from build123d import *

# Parameters (mm, degrees)
F0_W           = 70
F0_H           = 120
F0_R           = 6.5
F0_R_2         = 13
F1_DEPTH       = 5
F3_D           = 4.4
F3_DEPTH       = 10
F3_CSINK_D     = 8.96
F3_CSINK_ANGLE = 90
F3_TIP         = 1.3218933619
F4_R           = 5


# Not quite as in the source:
# - a feature names something its author has since deleted; it is built from what else it names


with BuildPart() as f1:
    # F0 (on Front) → F1 (new body)
    with BuildSketch(Plane.XZ):
        Rectangle(F0_W, F0_H)
        with Locations((0, -45)):
            Circle(F0_R, mode=Mode.SUBTRACT)
        Circle(F0_R_2, mode=Mode.SUBTRACT)
        with Locations((0, 45)):
            Circle(F0_R, mode=Mode.SUBTRACT)
    extrude(amount=F1_DEPTH)

    # F3
    with Locations(Plane.XZ.offset(5)):
        with Locations((14, 14), (-14, 14), (-14, -14), (14, -14)):
            CounterSinkHole(F3_D / 2, F3_CSINK_D / 2, depth=F3_DEPTH, counter_sink_angle=F3_CSINK_ANGLE)
            with Locations((0, 0, -(F3_DEPTH + F3_TIP / 2))):  # 118° drill point
                Cone(0, F3_D / 2, F3_TIP, mode=Mode.SUBTRACT)

    # F4
    f4_edges = [f1.edges().sort_by_distance(p)[0] for p in [
        (35, -2.5, 60),
        (35, -2.5, -60),
        (-35, -2.5, -60),
        (-35, -2.5, 60),
    ]]
    fillet(f4_edges, radius=F4_R)


solid = f1.part
Geometry check sheet. Reference: the model listing, model coordinates, mm. Coordinates: 2 decimals unless noted, no trailing zeros. Order: outer loops, then holes, each group sorted by start corner. A loop starts at its lowest first (then second) coordinate and runs counter-clockwise, first axis right, second up. Notation, with made-up numbers: (66.5, 73.5) - (99.5, 73.5) arc R14 ccw to (99.5, 88.5) - close; hole circle Ø5 at (21, 29). An arc over 180 degrees is marked (long way). Answer in a Markdown table with one row per item. Add a question column.
1) Gauge pin test, flat end, axial feed: P1, Ø1, axis at x = 26, z = -45.5, coming from the +Y side. Record the tip position at first contact, or that the pin passes through.
2) Cross-section at A-A, the plane z = 0. Record the cut outline in (x, y).
3) Release check for a two-part mould opening along X. For faces 1 (the flat face through (0, -2, 60)), 2 (the flat face through (-35, -2, -1)), 3 (the cylindrical face through (-16.032, -1.341, -14.843)), 4 (the conical face through (-13.499, -2.831, 11.744)) record: +X half, -X half, draft (parallel to the pull), parting line (faces both ways), or undercut.
4) Cross-section at C-C, the plane y = -1.95. Record the cut outline in (x, z).
5) Cross-section at B-B, the plane x = 0. Record the cut outline in (y, z).
6) Material ranges on line 1 along Z through (x, y) = (14, -1.3); line 2 along X through (y, z) = (-0.6, -14); line 3 along Z through (x, y) = (0, -3.5), recorded low to high. Write a range as [from, to].
7) Cross-section at D-D, the plane z = 45. Record the cut outline in (x, y), then the cut area to 3 significant figures.
Check result:
| question | item | result |
|---|---|---|
| 1 | P1 | stops at y = 0 |
| 2 | outline | (-35, -5) - (-13, -5) - (-13, 0) - (-35, 0) - close; (13, -5) - (35, -5) - (35, 0) - (13, 0) - close |
| 3 | face 1 | draft |
| 3 | face 2 | -X half |
| 3 | face 3 | undercut |
| 3 | face 4 | undercut |
| 4 | outline | (-35, -55) arc R5 ccw to (-30, -60) - (30, -60) arc R5 ccw to (35, -55) - (35, 55) arc R5 ccw to (30, 60) - (-30, 60) arc R5 ccw to (-35, 55) - close; hole circle Ø4.4 at (-14, -14); hole circle Ø4.4 at (-14, 14); hole circle Ø26 at (0, 0); hole circle Ø13 at (0, -45); hole circle Ø13 at (0, 45); hole circle Ø4.4 at (14, -14); hole circle Ø4.4 at (14, 14) |
| 5 | outline | (-5, -60) - (0, -60) - (0, -51.5) - (-5, -51.5) - close; (-5, -38.5) - (0, -38.5) - (0, -13) - (-5, -13) - close; (-5, 13) - (0, 13) - (0, 38.5) - (-5, 38.5) - close; (-5, 51.5) - (0, 51.5) - (0, 60) - (-5, 60) - close |
| 6 | line 1 | z = [-60, -16.2], [-11.8, 11.8], [16.2, 60] |
| 6 | line 2 | x = [-35, -16.2], [-11.8, 11.8], [16.2, 35] |
| 6 | line 3 | z = [-60, -51.5], [-38.5, -13], [13, 38.5], [51.5, 60] |
| 7 | outline | (-35, -5) - (-6.5, -5) - (-6.5, 0) - (-35, 0) - close; (6.5, -5) - (35, -5) - (35, 0) - (6.5, 0) - close |
| 7 | area | 285 mm² |
